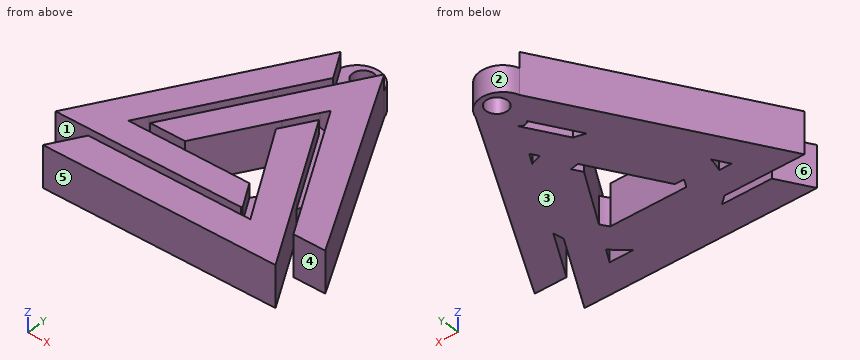
```python
from build123d import *

# Parameters (mm, degrees)
F1_DEPTH = 4.064
F2_DEPTH = 6.096
F0_R     = 1.5875
F3_DEPTH = 3.81


with BuildPart() as f1:
    # F0 (on Top) → F1 (new body)
    with BuildSketch(Plane.XY):
        with BuildLine():
            ThreePointArc((-3.332805, 6.675153), (-4.198232, 6.474047), (-5.045567, 6.206779))
            Line((-5.045567, 6.206779), (-12.475147, -6.74291))
            ThreePointArc((-12.475147, -6.74291), (-12.213975, -7.839217), (-11.84683, -8.904723))
            Line((-11.84683, -8.904723), (-6.879852, -8.904723))
            ThreePointArc((-6.879852, -8.904723), (-7.2945, -8.285602), (-7.642369, -7.626641))
            Line((-7.642369, -7.626641), (-11.558674, -7.626641))
            Line((-11.558674, -7.626641), (-3.332805, 6.675153))
        make_face()
        with BuildLine():
            ThreePointArc((10.060523, -7.176114), (10.205887, -6.419697), (10.300328, -5.655252))
            Line((10.300328, -5.655252), (3.436154, 5.922969))
            ThreePointArc((3.436154, 5.922969), (2.635064, 6.237061), (1.812747, 6.490423))
            Line((1.812747, 6.490423), (-0.487404, 2.481281))
            ThreePointArc((-0.487404, 2.481281), (0.148569, 2.391873), (0.773937, 2.245683))
            Line((0.773937, 2.245683), (2.580103, 5.393814))
            Line((2.580103, 5.393814), (10.060523, -7.176114))
        make_face()
        with BuildLine():
            Line((4.522967, -8.947072), (6.893241, -12.846554))
            ThreePointArc((6.893241, -12.846554), (7.344862, -12.378173), (7.769292, -11.885019))
            Line((7.769292, -11.885019), (5.257529, -7.752765))
            ThreePointArc((5.257529, -7.752765), (4.919634, -8.367992), (4.522967, -8.947072))
        make_face()
        with BuildLine():
            Line((6.756257, -12.978608), (-9.081211, -12.978608))
            ThreePointArc((-9.081211, -12.978608), (-8.44977, -13.534932), (-7.779364, -14.043628))
            Line((-7.779364, -14.043628), (5.45441, -14.043628))
            ThreePointArc((5.45441, -14.043628), (6.124816, -13.534932), (6.756257, -12.978608))
        make_face()
    extrude(amount=F1_DEPTH)

    # F0 (on Top) → F2 (join)
    with BuildSketch(Plane.XY):
        with BuildLine():
            Line((-1.438017, 12.494705), (-4.049945, 16.816666))
            Line((-4.049945, 16.816666), (-21.144284, -12.978608))
            Line((-21.144284, -12.978608), (-9.081211, -12.978608))
            Line((-9.081211, -12.978608), (6.756257, -12.978608))
            ThreePointArc((6.756257, -12.978608), (6.825022, -12.912864), (6.893241, -12.846554))
            Line((6.893241, -12.846554), (4.522967, -8.947072))
            Line((4.522967, -8.947072), (4.497225, -8.904723))
            Line((4.497225, -8.904723), (-6.879852, -8.904723))
            Line((-6.879852, -8.904723), (-11.84683, -8.904723))
            Line((-11.84683, -8.904723), (-13.715436, -8.904723))
            Line((-13.715436, -8.904723), (-12.475147, -6.74291))
            Line((-12.475147, -6.74291), (-5.045567, 6.206779))
            Line((-5.045567, 6.206779), (-1.438017, 12.494705))
        make_face()
        Polygon((19.434802, -12.978608), (2.500223, 16.816666), (0, 12.469688), (-3.332805, 6.675153), (-11.558674, -7.626641), (-7.642369, -7.626641), (-6.286587, -7.626641), (-0.487404, 2.481281), (1.812747, 6.490423), (2.445692, 7.59364), (3.436154, 5.922969), (10.300328, -5.655252), (14.641996, -12.978608), align=None)
        Polygon((5.45441, -14.043628), (-7.779364, -14.043628), (-15.313038, -14.043628), (-18.023162, -18.767349), (16.95852, -18.767349), (10.060523, -7.176114), (2.580103, 5.393814), (0.773937, 2.245683), (0, 0.896719), (5.257529, -7.752765), (7.769292, -11.885019), (9.081388, -14.043628), align=None)
    extrude(amount=F2_DEPTH)

    # F0 (on Top) → F3 (join)
    with BuildSketch(Plane.XY):
        with BuildLine():
            ThreePointArc((2.500223, 16.816666), (-0.774861, 19.287277), (-4.049945, 16.816666))
            Line((-4.049945, 16.816666), (-1.438017, 12.494705))
            ThreePointArc((-1.438017, 12.494705), (-0.725922, 12.084814), (0, 12.469688))
            Line((0, 12.469688), (2.500223, 16.816666))
        make_face()
        with Locations((-0.774861, 16.946895)):
            Circle(F0_R, mode=Mode.SUBTRACT)
    extrude(amount=F3_DEPTH)


solid = f1.part
```
Geometry: final body of the model. Coordinates: model frame, mm. Face numbers are marked on the shaded views. A direction names the side the tool comes from. Coordinates: 2 decimals unless noted, no trailing zeros. Order: outer loops, then holes, each group sorted by start corner. A loop starts at its lowest first (then second) coordinate and runs counter-clockwise, first axis right, second up. Notation, with made-up numbers: M -27,63.25 L 6,63.25 A17 ccw 6,70.25 Z; hole C 40.5,80 d8. An arc over 180 degrees is marked long. Answer in a Markdown table with one row per item. Add a question column.
Q1. Reachability of the marked faces 4, 5 and 6 from +Z, -Z, +X, -X, +Y, -Y: full face, straight path, thin tool, end or side. Return the list, or none.
Q2. Section query A-A on x = -17. Return the cut outline in (y, z).
Q3. Section query C-C on y = -13.5. Return the cut outline in (x, z), and give its area (3 significant figures).
Q4. Section query D-D on z = 0.75. Count the separate pieces of the cut face and the enclosed holes in it, and give its area (3 significant figures).
Q5. Mould query, pull axis Y, two halves, no side actions, for the marked faces 1, 2 and 3. Classes: released by +Y, released by -Y, zero draft, split by the parting line, or undercut.
Q6. Contact query for flat-ended pins moving along their axis: P1, Ø0.5, axis at x = -4.5, y = -13.5, coming from the +Z side; P2, Ø3, axis at x = -3.5, z = 2, coming from the +Y side; P3, Ø2, axis at y = -8, z = 4, coming from the +X side; P4, Ø2.5, axis at x = -0.77, y = 16.95, coming from the -Z side. Output: stop coordinate, or through.
Q7. Line query: L1, parallel to X at y = -12, z = 3.25; L2, parallel to Y at x = -13, z = 4.25; L3, parallel to Y at x = -10, z = 5.5. Output: solid intervals per line, ascending.
Q8. Section query B-B on y = 1.5. Return the cut outline in (x, z), and give its area (3 significant figures).
Completed:
| question | item | result |
|---|---|---|
| 1 | face 4 | +Z, -Z, +X |
| 1 | face 5 | +Z, -Z, +X, -X, -Y |
| 1 | face 6 | +Z, -Z, -X |
| 2 | outline | M -18.77,0 L -16.98,0 L -16.98,6.1 L -18.77,6.1 Z; M -12.98,0 L -5.76,0 L -5.76,6.1 L -12.98,6.1 Z |
| 3 | outline | M -8.49,0 L 6.17,0 L 6.17,4.06 L -8.49,4.06 Z; M 8.75,0 L 13.82,0 L 13.82,6.1 L 8.75,6.1 Z |
| 3 | area | 90.5 mm2 |
| 4 | separate pieces | 1 |
| 4 | enclosed holes | 6 |
| 4 | area | 787 mm2 |
| 5 | face 1 | undercut |
| 5 | face 2 | released by +Y |
| 5 | face 3 | zero draft |
| 6 | P1 | stops at z = 4.06 |
| 6 | P2 | stops at y = 19.06 |
| 6 | P3 | stops at x = 17.17 |
| 6 | P4 | passes through |
| 7 | L1 | x = -20.58 to 7.67, 7.84 to 12.93, 14.06 to 18.88 |
| 7 | L2 | y = -18.77 to -14.04, -12.98 to -8.9, -7.66 to 1.22 |
| 7 | L3 | y = -18.77 to -14.04, -12.98 to -8.9, -7.63 to -4.92, -2.43 to 6.45 |
| 8 | outline | M -12.84,0 L -1.05,0 L -1.05,6.1 L -6.31,6.1 L -6.31,4.06 L -7.75,4.06 L -7.75,6.1 L -12.84,6.1 Z; M 0.35,0 L 11.21,0 L 11.21,6.1 L 6.06,6.1 L 6.06,4.06 L 4.9,4.06 L 4.9,6.1 L 0.35,6.1 Z |
| 8 | area | 133 mm2 |
